Read the model definition and answer for the solid it produces. Units are mm, in the model's axes. A direction names the side the tool comes from. Coordinates: 2 decimals unless noted, no trailing zeros. Order: outer loops, then holes, each group sorted by start corner. A loop starts at its lowest first (then second) coordinate and runs counter-clockwise, first axis right, second up. Notation, with made-up numbers: (48.25, 44) - (57.25, 44) arc R14 ccw to (57.25, 53) - close; hole circle Ø7 at (25, 18.5). An arc over 180 degrees is marked (long way). Use one line per item in the form item = value. Start each with the question number.
from build123d import *

# Parameters (mm, degrees)
BOSS_EXTRUDE1_DEPTH = 5
SKETCH2_W           = 17.35
SKETCH2_H           = 13
BOSS_EXTRUDE2_DEPTH = 5


with BuildPart() as part:
    # Sketch1 → Boss-Extrude1 (new body)
    with BuildSketch(Plane.XY):
        with BuildLine():
            Line((0, 0), (0, -85))
            Line((0, -85), (-41.280574715, -85))
            ThreePointArc((-41.280574715, -85), (-92.819395035, -57.855339059), (-99.590093663, 0))
            Line((-99.590093663, 0), (0, 0))
        make_face()
    extrude(amount=BOSS_EXTRUDE1_DEPTH)

    # Sketch2 → Boss-Extrude2 (add)
    with BuildSketch(Plane.XY.offset(5)):
        with Locations((-8.675, -91.5)):
            Rectangle(SKETCH2_W, SKETCH2_H)
    extrude(amount=-BOSS_EXTRUDE2_DEPTH)


solid = part.part
Q1. Consider probe 1 along X at (y, z) = (-23.5, 3.75); probe 2 along Y at (x, z) = (-34, 4.8); probe 3 along X at (y, z) = (-92, 1.2). Determine where each line is inside the solid, lowest interval first.
Q2. Which of the six approach directions +Z, -Z, +X, -X, +Y, -Y give full straight-line access (tool end or side, diameter ignored) to faces 1 (the flat face through (-53, -37, 0)), 2 (the flat face through (-29, -85, 2))?
Q3. A cutting plane is placed at B-B (z = 4.2). Give the vertices of the cut face in (x, y).
Q4. Given P1, Ø1.5, axis at y = -66.5, z = 4, coming from the +X side, flat-ended and moving along its own axis, determine where the tip first touches the part or whether it passes through.
Q5. A cutting plane is placed at C-C (x = -27.5). Give the vertices of the cut face in (y, z).
Q6. A cutting plane is placed at A-A (y = -91). Give the vertices of the cut face in (x, z), then the cut area to 4 significant figures.
Result sheet:
q1.probe_1 = -103.77 to 0
q1.probe_2 = -85 to 0
q1.probe_3 = -17.35 to 0
q2.face_1 = -Z, +X, -X, +Y, -Y
q2.face_2 = +Z, -Z, -X, -Y
q3.outline = (-99.59, 0) arc R62.5 ccw to (-41.28, -85) - (-17.35, -85) - (-17.35, -98) - (0, -98) - (0, 0) - close
q4.P1 = 0
q5.outline = (-85, 0) - (0, 0) - (0, 5) - (-85, 5) - close
q6.outline = (-17.35, 0) - (0, 0) - (0, 5) - (-17.35, 5) - close
q6.area = 86.75 mm^2
